```python
from build123d import *

# Parameters (mm, degrees)
MODEL_R                 = 6
MODEL_R_2               = 8
MODEL_W                 = 32
MODEL_H                 = 32
SALIENTE_EXTRUIR1_DEPTH = 3


with BuildPart() as part:
    # Model → Saliente-Extruir1 (new body)
    with BuildSketch(Plane.XY):
        Polygon((18.582508913, 92.133016607), (18.582508913, -27.866983393), (2.582508913, -27.866983393), (2.582508913, -57.866983393), (-1.417491087, -57.866983393), (-3.417491087, -52.866983393), (-1.417491087, -52.866983393), (-1.417491087, -49.866983393), (-17.417491087, -49.866983393), (-17.417491087, -52.866983393), (-15.417491087, -52.866983393), (-17.417491087, -57.866983393), (-21.417491087, -57.866983393), (-21.417491087, -27.866983393), (-37.417491087, -27.866983393), (-37.417491087, 92.133016607), align=None)
        with Locations((-9.417491087, 57.433016607)):
            Circle(MODEL_R, mode=Mode.SUBTRACT)
        with Locations((-22.417491087, 76.633016607)):
            Circle(MODEL_R_2, mode=Mode.SUBTRACT)
        with Locations((3.582508913, 76.633016607)):
            Circle(MODEL_R_2, mode=Mode.SUBTRACT)
        with Locations((-9.417491087, 26.433016607)):
            Rectangle(MODEL_W, MODEL_H, mode=Mode.SUBTRACT)
    extrude(amount=SALIENTE_EXTRUIR1_DEPTH)


solid = part.part
```
Work out the finished part from the listing and answer in its coordinate system (mm). A direction names the side the tool comes from. Coordinates: 2 decimals unless noted, no trailing zeros. Order: outer loops, then holes, each group sorted by start corner. A loop starts at its lowest first (then second) coordinate and runs counter-clockwise, first axis right, second up. Notation, with made-up numbers: M -12.75,45.5 L -1.75,45.5 A24 ccw -1.75,65.5 Z; hole C 28,-17.75 d5. An arc over 180 degrees is marked long. Use CSV: the item, a comma, the result in double quotes.
1) Section D-D on x = 8 is taken. Write down the section's boundary in (y, z).
Worked out:
outline,"M -27.87,0 L 69.96,0 L 69.96,3 L -27.87,3 Z; M 83.3,0 L 92.13,0 L 92.13,3 L 83.3,3 Z"
2) Flat-ended cylindrical pins translate along their axes: pin 1 Ø5 at (x, y) = (2.5, 58.5) entering from -Z; pin 2 Ø1.5 at (y, z) = (-51, 2) entering from -X; pin 3 Ø0.9 at (x, z) = (11, 2) entering from -Y; pin 4 Ø1.5 at (y, z) = (-52, 2) entering from +X. Find the tip coordinate at first contact, or state that the pin passes through.
Worked out:
pin 1,"stops at z = 0"
pin 2,"stops at x = -21.42"
pin 3,"stops at y = -27.87"
pin 4,"stops at x = 2.58"
3) For faces 5 (the face through (10, 35, 3)), 6 (the face through (-1.417, -51, 1)), 7 (the face through (-29, -27.867, 1)), 8 (the face through (-2.403, -55.402, 1.479)), 9 (the face through (11, -27.867, 1)), determine the directions among +Z, -Z, +X, -X, +Y, -Y from which every point of the face is accessible in a straight line to the end or side of a thin tool.
Worked out:
face 5,"+Z, +X, -X, +Y, -Y"
face 6,"+Z, -Z"
face 7,"+Z, -Z, -X, -Y"
face 8,"+Z, -Z, -Y"
face 9,"+Z, -Z, +X, -Y"
4) Section C-C on z = 0.5 is taken. Write down the section's boundary in (x, y), plus the area to 3 significant figures.
Worked out:
outline,"M -37.42,-27.87 L -21.42,-27.87 L -21.42,-57.87 L -17.42,-57.87 L -15.42,-52.87 L -17.42,-52.87 L -17.42,-49.87 L -1.42,-49.87 L -1.42,-52.87 L -3.42,-52.87 L -1.42,-57.87 L 2.58,-57.87 L 2.58,-27.87 L 18.58,-27.87 L 18.58,92.13 L -37.42,92.13 Z; hole C -22.42,76.63 d16; hole M -25.42,10.43 L 6.58,10.43 L 6.58,42.43 L -25.42,42.43 Z; hole C -9.42,57.43 d12; hole C 3.58,76.63 d16"
area,"5,780 mm^2"
5) Section B-B on x = -13 is taken. Write down the section's boundary in (y, z), plus the area to 3 significant figures.
Worked out:
outline,"M -49.87,0 L 10.43,0 L 10.43,3 L -49.87,3 Z; M 42.43,0 L 52.62,0 L 52.62,3 L 42.43,3 Z; M 62.25,0 L 92.13,0 L 92.13,3 L 62.25,3 Z"
area,"301 mm^2"
6) Section A-A on y = 30.5 is taken. Write down the section's boundary in (x, z), plus the area to 3 significant figures.
Worked out:
outline,"M -37.42,0 L -25.42,0 L -25.42,3 L -37.42,3 Z; M 6.58,0 L 18.58,0 L 18.58,3 L 6.58,3 Z"
area,"72.0 mm^2"
7) Consider line 1 (X direction, y = 76, z = 1.85); line 2 (X direction, y = 83.5, z = 0.85); line 3 (Y direction, x = -6.5, z = 0.3). Determine where each line is inside the solid, lowest interval first. Write a range as [from, to].
Worked out:
line 1,"x = [-37.42, -30.39], [-14.44, -4.39], [11.56, 18.58]"
line 2,"x = [-37.42, -26.52], [-18.31, -0.52], [7.69, 18.58]"
line 3,"y = [-49.87, 10.43], [42.43, 52.19], [62.68, 92.13]"
8) Determine the mould class of faces 1 (the face through (-10, 42.433, 1)), 2 (the face through (10, 35, 0)), 3 (the face through (-21.417, -43, 1)), 4 (the face through (-9, -49.867, 1)) for opening direction X: released by +X, released by -X, zero draft, split by the parting line, or undercut.
Worked out:
face 1,"undercut"
face 2,"zero draft"
face 3,"released by -X"
face 4,"undercut"
